Source: three-view drawing plus pictorial views. Frame: mm from the lowest corner of the part. A direction names the side the tool comes from. Give positions to 0.01 mm unless a question says otherwise; leave off trailing zeros. Order: outer loops, then holes, each group sorted by start corner. A loop starts at its lowest first (then second) coordinate and runs counter-clockwise, first axis right, second up.
1) Section C-C, the plane y = 28. Return loops of the section in (x, z), plus the area to 3 significant figures.
2) Access query for the marked faces 1 and 2. Directions: +Z, -Z, +X, -X, +Y, -Y. A direction counts if a zero-diameter tool reaches every point of the face in a straight line with its end or side. Return the directions, or none.
3) Section B-B, the plane z = 75. Return loops of the section in (x, y).
4) Material intervals for line 1 (X direction, y = 26.25, z = 95); line 2 (X direction, y = 19.25, z = 75); line 3 (X direction, y = 27.25, z = 94), sorted ascending.
5) First-contact query: P1, Ø6, axis at x = 86, z = 61, coming from the -Y side; P2, Ø3, axis at x = 90, z = 55, coming from the -Y side; P3, Ø8, axis at x = 60, z = 55, coming from the +Y side; P4, Ø4, axis at y = 23, z = 87.5, coming from the +X side. Flat tips, straight axial feed; report the tip coordinate or a pass-through.
6) Section A-A, the plane x = 75. Return loops of the section in (y, z).
7) Section D-D, the plane x = 60. Return loops of the section in (y, z).
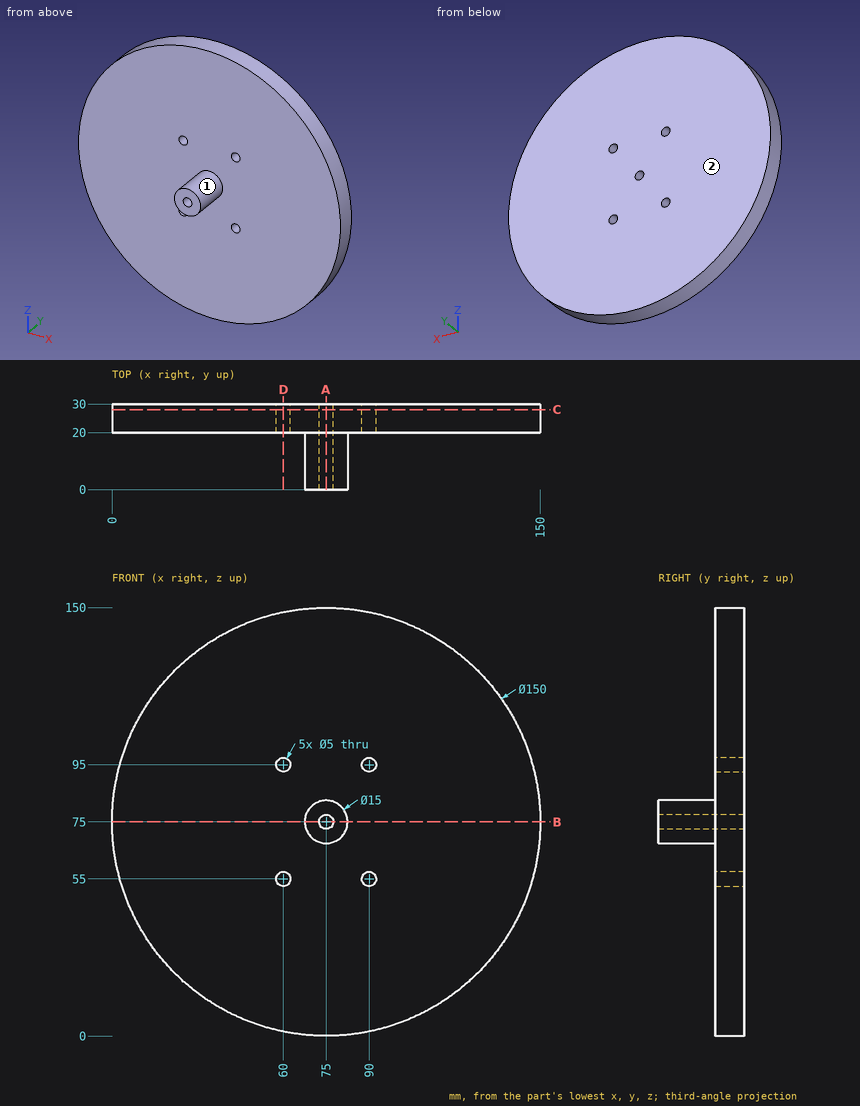
From the geometry:
1. outline: circle Ø150 at (75, 75); hole circle Ø5 at (60, 55); hole circle Ø5 at (60, 95); hole circle Ø5 at (75, 75); hole circle Ø5 at (90, 55); hole circle Ø5 at (90, 95)
1. area: 17,600 mm2
2. face 1: -Y
2. face 2: +Z, -Z, +X, -X, +Y
3. outline: (0, 20) - (67.5, 20) - (67.5, 0) - (72.5, 0) - (72.5, 30) - (0, 30) - close; (77.5, 0) - (82.5, 0) - (82.5, 20) - (150, 20) - (150, 30) - (77.5, 30) - close
4. line 1: x = 2.72 to 57.5, 62.5 to 87.5, 92.5 to 147.28
4. line 2: x = 67.5 to 72.5, 77.5 to 82.5
4. line 3: x = 2.45 to 57.71, 62.29 to 87.71, 92.29 to 147.55
5. P1: stops at y = 20
5. P2: passes through
5. P3: stops at y = 30
5. P4: stops at x = 149.26
6. outline: (0, 67.5) - (20, 67.5) - (20, 0) - (30, 0) - (30, 72.5) - (0, 72.5) - close; (0, 77.5) - (30, 77.5) - (30, 150) - (20, 150) - (20, 82.5) - (0, 82.5) - close
7. outline: (20, 1.52) - (30, 1.52) - (30, 52.5) - (20, 52.5) - close; (20, 57.5) - (30, 57.5) - (30, 92.5) - (20, 92.5) - close; (20, 97.5) - (30, 97.5) - (30, 148.48) - (20, 148.48) - close
